Part model, mm, in its own coordinate system. A direction names the side the tool comes from. Round coordinates to 2 decimals unless told otherwise and drop trailing zeros. Loops run counter-clockwise (first coordinate to the right, second up) from the corner with the lowest first, then second, coordinate; pieces in that order, holes last. Notation, with made-up numbers: (72, -1.5) -> (117, -1.5) arc R24 cw to (117, 16.5) -> close; hole circle Ø2 at (-11, -21). An arc over 180 degrees is marked (long way). Use a Markdown table: item, result. Add a question column.
Item 1: Cut at D-D, the plane y = 27.5. List the corners of the cut face in (x, z), plus the area to 3 significant figures.
Item 2: Which spindle directions (+Z, -Z, +X, -X, +Y, -Y) get a long thin tool onto all of the face, cutting with end or side? Do faces 1 (the face through (0, 12, -12)), 2 (the face through (-8, 87, -9)), 3 (the face through (-12, 55, 0)). Say none if no direction does.
Item 3: Two-plate mould, pull along X, no slides. Class faces 4 (the face through (0, 12, 12)), 5 (the face through (2.17, 104.86, 9.76)), 6 (the face through (-2.17, -9.76, -19.4)), 7 (the face through (-8, 87, 9)): pulls with the +X half, pulls with the -X half, needs draft (parallel to the pull), parting line crosses it, or undercut.
Item 4: Cut at A-A, the plane x = 0. State how many separate pieces and enclosed holes the cut face has, plus the area to 3 significant figures.
Item 5: Cut at C-C, the plane z = 0. List the corners of the cut face in (x, y).
Item 6: Flat gauge pins, fed straight in: pin 1 (2 mm diameter, centred on x = 1.5, z = -3, fed in from -Y); pin 2 (4 mm diameter, centred on y = 7.5, z = 13.5, fed in from +X); pin 3 (6 mm diameter, centred on x = -12, z = -6.5, fed in from -Y); pin 4 (4 mm diameter, centred on x = 15.5, z = -2, fed in from +Y). Where does each tip first touch, or does it go through?
Item 7: Probe line 1 (X direction, y = 0, z = 22.75); line 2 (Z direction, x = -11, y = -2.5); line 3 (Y direction, x = -8.5, z = -15). List the from-to ranges inside material, lowest first. Write a range as [from, to].
Item 8: Cut at B-B, the plane y = 0. List the corners of the cut face in (x, z).
Solid Edge part; units mm, degrees
sketch "Sketch1" plane through (0, 0, 0) normal (0, 0, 1) x (1, 0, 0)
  circle A0 centre (0, 0) radius 20
  circle A1 centre (0, 0) radius 10
extrude "Protrusion1" add sketch "Sketch1" along normal mid plane 54
sketch "Sketch2" plane through (0, 0, 0) normal (0, -1, 0) x (1, 0, 0)
  line L0 (-20, 12) -> (20, 12)
  line L1 (20, 12) -> (20, -12)
  line L2 (20, -12) -> (-20, -12)
  line L3 (-20, -12) -> (-20, 12)
  dimension "D1" = 20
  dimension "D2" = 20
extrude "ExtrudedCutout_1" cut sketch "Sketch2" along normal mid plane 239.353
sketch "Sketch3" plane through (0, 0, 0) normal (1, 0, 0) x (0, 1, 0)
  line L0 (24, 12) -> (20, 12)
  line L1 (12, 12) -> (20, 12)
  line L2 (12, 24) -> (12, 12)
  line L3 (24, 24) -> (12, 24)
  line L4 (24, -24) -> (12, -24)
  line L5 (12, -24) -> (12, -12)
  line L6 (12, -12) -> (20, -12)
  line L7 (24, -12) -> (20, -12)
  arc A0 (24, 24) -> (24, -24) centre (24, 0) cw
  arc A1 (24, -12) -> (24, 12) centre (24, 0) ccw
extrude "ExtrudedProtrusion_2" add sketch "Sketch3" along normal mid plane 24
sketch "Sketch4" plane through (0, 95, 0) normal (0, -1, 0) x (1, 0, 0)
  line L0 (-12, 12) -> (12, 12)
  line L1 (12, 12) -> (12, -12)
  line L2 (12, -12) -> (-12, -12)
  line L3 (-12, -12) -> (-12, 12)
  dimension "D1" = 12
  dimension "D2" = 12
extrude "Protrusion2" add sketch "Sketch4" along normal up to next
sketch "Sketch5" plane through (0, 95, 0) normal (0, 1, 0) x (-1, 0, 0)
  circle A0 centre (0, 0) radius 10
extrude "ExtrudedProtrusion_4" add sketch "Sketch5" along normal blind 20
fillet "Round_1" radius 15 2 edges at (0, 44.7846, 12) (0, 44.7846, -12)
sketch "Sketch6" plane through (0, 95, 0) normal (0, 1, 0) x (-1, 0, 0)
  line L0 (12, 5) -> (12, -5)
  line L1 (5, 12) -> (12, 5)
  line L2 (-5, 12) -> (5, 12)
  line L3 (-12, 5) -> (-5, 12)
  line L4 (-12, -5) -> (-12, 5)
  line L5 (-12, -5) -> (-5, -12)
  line L6 (-5, -12) -> (5, -12)
  line L7 (5, -12) -> (12, -5)
extrude "ExtrudedCutout_3" cut sketch "Sketch6" against normal blind 20 flip side to cut
fillet "Round_2" radius 4 4 edges at (8.5, 75, 8.5) (-8.5, 75, 8.5) (-8.5, 75, -8.5) (8.5, 75, -8.5)
properties part number "1"
A:
| question | item | result |
|---|---|---|
| 1 | outline | (-12, -23.74) -> (12, -23.74) -> (12, -11.48) -> (-12, -11.48) -> close; (-12, 11.48) -> (12, 11.48) -> (12, 23.74) -> (-12, 23.74) -> close |
| 1 | area | 589 mm^2 |
| 2 | face 1 | +X, -X, -Y |
| 2 | face 2 | -Z, -X, +Y |
| 2 | face 3 | +Z, -Z, -X, +Y |
| 3 | face 4 | needs draft |
| 3 | face 5 | parting line crosses it |
| 3 | face 6 | undercut |
| 3 | face 7 | pulls with the -X half |
| 4 | separate pieces | 3 |
| 4 | enclosed holes | 0 |
| 4 | area | 2,940 mm^2 |
| 5 | outline | (-12, 36) -> (12, 36) -> (12, 95) -> (10, 95) -> (10, 115) -> (-10, 115) -> (-10, 95) -> (-12, 95) -> close |
| 6 | pin 1 | stops at y = 35.31 |
| 6 | pin 2 | stops at x = 19.23 |
| 6 | pin 3 | stops at y = 31.33 |
| 6 | pin 4 | passes through |
| 7 | line 1 | x = [-20, -10], [10, 20] |
| 7 | line 2 | z = [-27, -12], [12, 27] |
| 7 | line 3 | y = [-18.1, -5.27], [5.27, 43.14] |
| 8 | outline | (-20, -27) -> (-10, -27) -> (-10, -12) -> (-20, -12) -> close; (-20, 12) -> (-10, 12) -> (-10, 27) -> (-20, 27) -> close; (10, -27) -> (20, -27) -> (20, -12) -> (10, -12) -> close; (10, 12) -> (20, 12) -> (20, 27) -> (10, 27) -> close |
